Design review of the part built by this model. Coordinates are the model's own, in mm. Face numbers are marked on the shaded views. A direction names the side the tool comes from. Coordinates: 2 decimals unless noted, no trailing zeros. Order: outer loops, then holes, each group sorted by start corner. A loop starts at its lowest first (then second) coordinate and runs counter-clockwise, first axis right, second up. Notation, with made-up numbers: M -19.75,76.5 L -7.75,76.5 A17 cw -7.75,104.5 Z; hole C 85,52 d11. An arc over 180 degrees is marked long. Answer as a JSON object with one key per item and string values.
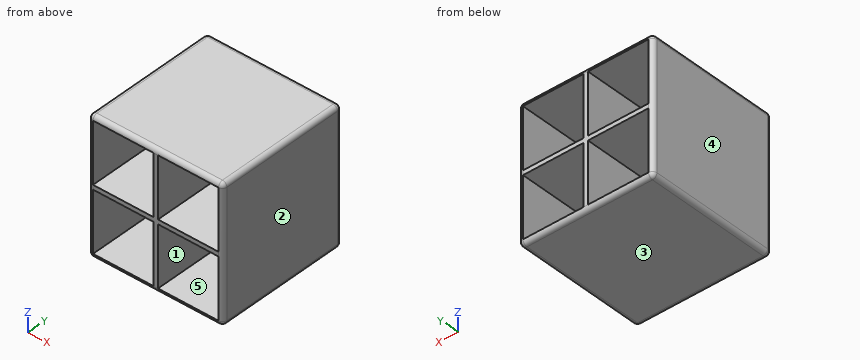
from build123d import *

# Parameters (mm, degrees)
F0_W     = 150
F0_H     = 150
F0_W_2   = 67.5
F0_H_2   = 67.5
F1_DEPTH = 150
F2_R     = 5
F3_R     = 4.99999


# Not quite as in the source:
# - a fillet or chamfer is up to 0.001 mm smaller than in the source, because OpenCascade refuses the exact size


with BuildPart() as f1:
    # F0 (on Front) → F1 (new body)
    with BuildSketch(Plane.XZ):
        with Locations((75, 75)):
            Rectangle(F0_W, F0_H)
        with Locations((38.75, 38.75)):
            Rectangle(F0_W_2, F0_H_2, mode=Mode.SUBTRACT)
        with Locations((111.25, 38.75)):
            Rectangle(F0_W_2, F0_H_2, mode=Mode.SUBTRACT)
        with Locations((38.75, 111.25)):
            Rectangle(F0_W_2, F0_H_2, mode=Mode.SUBTRACT)
        with Locations((111.25, 111.25)):
            Rectangle(F0_W_2, F0_H_2, mode=Mode.SUBTRACT)
    extrude(amount=F1_DEPTH)

    # F2
    f2_edges = [f1.edges().sort_by_distance(p)[0] for p in [
        (150, -75, 150),
    ]]
    fillet(f2_edges, radius=F2_R)

    # F3 (radius 5 in the source; OpenCascade refuses exactly that, so slightly less here)
    f3_edges = [f1.edges().sort_by_distance(p)[0] for p in [
        (72.5, -150, 150),
        (150, -150, 72.5),
        (72.5, 0, 150),
        (0, -75, 150),
        (75, -150, 0),
        (150, -75, 0),
        (0, -150, 75),
        (150, 0, 72.5),
        (0, 0, 75),
        (0, -75, 0),
        (75, 0, 0),
    ]]
    fillet(f3_edges, radius=F3_R)


solid = f1.part
1) Add section C-C (y = -76.5). State the section outline as (x, z) points, and give its area (3 significant figures).
Taken from the geometry:
{"outline": "M 0,5 A5 ccw 5,0 L 145,0 A5 ccw 150,5 L 150,145 A5 ccw 145,150 L 5,150 A5 ccw 0,145 Z; hole M 5,5 L 72.5,5 L 72.5,72.5 L 5,72.5 Z; hole M 5,77.5 L 72.5,77.5 L 72.5,145 L 5,145 Z; hole M 77.5,5 L 145,5 L 145,72.5 L 77.5,72.5 Z; hole M 77.5,77.5 L 145,77.5 L 145,145 L 77.5,145 Z", "area": "4,250 mm2"}
2) Add section A-A (z = 62). Count the separate pieces of the cut face and the enclosed holes in it, and give its area (3 significant figures).
Taken from the geometry:
{"separate pieces": "3", "enclosed holes": "0", "area": "2,230 mm2"}
3) Tool access review of the marked faces 4 and 5: name each direction out of +Z, -Z, +X, -X, +Y, -Y from which nothing blocks a thin tool from reaching the whole face with its end or side.
Taken from the geometry:
{"face 4": "+Z, -Z, -X, +Y, -Y", "face 5": "+Y, -Y"}
4) To check wall thickness, follow L1, parallel to X at y = -102, z = 62.5. State the ranges of the line that lie inside material, in increasing order.
Taken from the geometry:
{"L1": "x = 0 to 5, 72.5 to 77.5, 145 to 150"}
5) Mouldability with a two-part tool opening along X and no side actions: class the marked faces 1, 2 and 3 as released by +X, released by -X, zero draft, split by the parting line, or undercut.
Taken from the geometry:
{"face 1": "undercut", "face 2": "released by +X", "face 3": "zero draft"}
6) Insertion check: pin 1 Ø6 at (x, z) = (79, 95.5) entering from -Y. The pin has a flat end and moves straight along its axis. Give the tip position at first contact, or say it passes through.
Taken from the geometry:
{"pin 1": "stops at y = -150"}
